Can you work these out from the model? Positions are in its coordinate system, mm. A direction names the side the tool comes from. Give positions to 0.01 mm unless a question says otherwise; leave off trailing zeros. Loops run counter-clockwise (first coordinate to the right, second up) from the corner with the lowest first, then second, coordinate; pieces in that order, holes last. Notation, with made-up numbers: (27, 81.25) - (54, 81.25) arc R19 ccw to (54, 102.25) - close; hole circle Ø2 at (44.5, -28.5). An arc over 180 degrees is marked (long way). Answer in a Markdown table with one row per item.
from build123d import *

# Parameters (mm, degrees)
SKETCH1_W           = 9
SKETCH1_H           = 1
SKETCH1_W_2         = 1
SKETCH1_H_2         = 9
BOSS_EXTRUDE1_DEPTH = 50


with BuildPart() as part:
    # Sketch1 → Boss-Extrude1 (new body)
    with BuildSketch(Plane(origin=(0, 0, 0), x_dir=(0, 0, -1), z_dir=(1, 0, 0))):
        with Locations((-15.137894846, 6.81112979)):
            Rectangle(SKETCH1_W, SKETCH1_H)
        with Locations((-10.137894846, 11.81112979)):
            Rectangle(SKETCH1_W_2, SKETCH1_H_2)
        with BuildLine():
            Line((-9.637894846, 7.31112979), (-10.637894846, 7.31112979))
            Line((-10.637894846, 7.31112979), (-10.637894846, 6.31112979))
            Line((-10.637894846, 6.31112979), (-10.137894846, 6.31112979))
            ThreePointArc((-10.137894846, 6.31112979), (-9.784341456, 6.4575764), (-9.637894846, 6.81112979))
            Line((-9.637894846, 6.81112979), (-9.637894846, 7.31112979))
        make_face()
    extrude(amount=BOSS_EXTRUDE1_DEPTH)


solid = part.part
Q1. On a 3-axis mill with a long thin cutter (end or side, diameter ignored), from which of +Z, -Z, +X, -X, +Y, -Y can I reach the whole of each face in a straight line? I mean faces 1 (the face through (0, 7, 12)), 2 (the face through (25, 7.311, 15)). Say none if no direction works.
Checked values:
| item | result |
|---|---|
| face 1 | +Z, -Z, -X, +Y, -Y |
| face 2 | +Z, +X, -X, +Y |
Q2. Imagine slicing it at B-B, the plane z = 12.75. Write out the boundary of the cut face in (x, y), and give its area (3 significant figures).
Checked values:
| item | result |
|---|---|
| outline | (0, 6.31) - (50, 6.31) - (50, 7.31) - (0, 7.31) - close |
| area | 50.0 mm² |
Q3. For pin 1 (2.5 mm diameter, centred on x = 36, z = 15.5, fed in from +Y); pin 2 (3 mm diameter, centred on y = 9.5, z = 14, fed in from +X), each with a flat end and sliding along its axis, tell me the tip position at first contact or that it passes through.
Checked values:
| item | result |
|---|---|
| pin 1 | stops at y = 7.31 |
| pin 2 | passes through |
Q4. If I drill on line 1 (Y direction, x = 32.5, z = 15.75); line 2 (Z direction, x = 39.5, y = 10.75); line 3 (Y direction, x = 15, z = 10), over which ranges is the centre line in solid material (lowest first)? Write a range as [from, to].
Checked values:
| item | result |
|---|---|
| line 1 | y = [6.31, 7.31] |
| line 2 | z = [9.64, 10.64] |
| line 3 | y = [6.33, 16.31] |
Q5. Imagine slicing it at C-C, the plane y = 9. Write out the boundary of the cut face in (x, z).
Checked values:
| item | result |
|---|---|
| outline | (0, 9.64) - (50, 9.64) - (50, 10.64) - (0, 10.64) - close |
Q6. Imagine slicing it at A-A, the plane x = 26. Write out the boundary of the cut face in (y, z).
Checked values:
| item | result |
|---|---|
| outline | (6.31, 10.14) arc R0.5 ccw to (6.81, 9.64) - (16.31, 9.64) - (16.31, 10.64) - (7.31, 10.64) - (7.31, 19.64) - (6.31, 19.64) - close |
